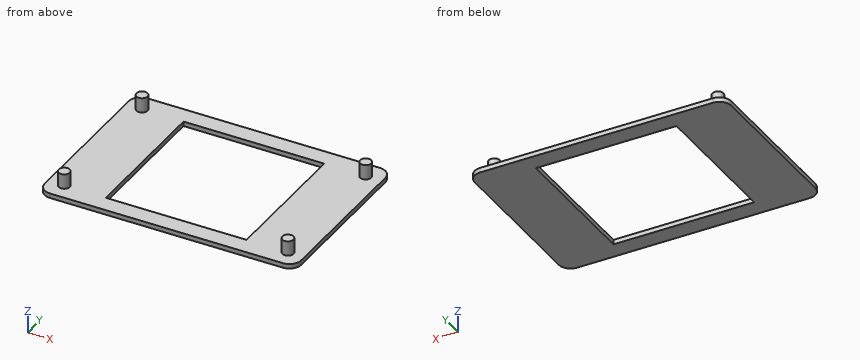
from build123d import *

# Parameters (mm, degrees)
SKETCH1_W           = 109.3978
SKETCH1_H           = 75
BOSS_EXTRUDE1_DEPTH = 2
SKETCH2_R           = 2.375
BOSS_EXTRUDE2_DEPTH = 6.35
CUT_EXTRUDE1_REACH  = 4
SKETCH3_W           = 60
SKETCH3_H           = 60
FILLET1_R           = 5


with BuildPart() as part:
    # Sketch1 → Boss-Extrude1 (new body)
    with BuildSketch(Plane.XY):
        with Locations((54.6989, 37.5)):
            Rectangle(SKETCH1_W, SKETCH1_H)
    extrude(amount=BOSS_EXTRUDE1_DEPTH)

    # Sketch2 → Boss-Extrude2 (add)
    with BuildSketch(Plane.XY.offset(2)):
        with Locations((6.9977, 67.4974)):
            Circle(SKETCH2_R)
        with Locations((102.4001, 67.4974)):
            Circle(SKETCH2_R)
        with Locations((102.4001, 7.5026)):
            Circle(SKETCH2_R)
        with Locations((6.9977, 7.5026)):
            Circle(SKETCH2_R)
    extrude(amount=BOSS_EXTRUDE2_DEPTH)

    # Sketch3 → Cut-Extrude1 (cut, up to next)
    with BuildSketch(Plane.XY.offset(2), mode=Mode.PRIVATE) as cut_extrude1_sk1:
        with Locations((54.6989, 37.5)):
            Rectangle(SKETCH3_W, SKETCH3_H)
    cut_extrude1_tool1 = extrude(cut_extrude1_sk1.sketch, amount=-CUT_EXTRUDE1_REACH, mode=Mode.PRIVATE) & part.part
    add(cut_extrude1_tool1.solids().sort_by_distance((54.6989, 37.5, 2))[0], mode=Mode.SUBTRACT)

    # Fillet1
    fillet1_edges = [part.edges().sort_by_distance(p)[0] for p in [
        (0, 75, 1),
        (109.3978, 75, 1),
        (109.3978, 0, 1),
        (0, 0, 1),
    ]]
    fillet(fillet1_edges, radius=FILLET1_R)


solid = part.part
CAD build for the part. Positions are in the model's coordinates, mm. Coordinates: 2 decimals unless noted, no trailing zeros. Write each loop counter-clockwise with the first axis right and the second up, starting at its lowest first coordinate (ties: lowest second). Pieces come first, ordered by that corner, then holes. Notation, with made-up numbers: (62.5, -0.75) - (70.5, -0.75) arc R32 ccw to (70.5, 38.25) - close; hole circle Ø5 at (14.25, 84). An arc over 180 degrees is marked (long way). Use a Markdown table: item, result. Add a question column.
Item 1: Band-saw the part on C-C, the plane x = 101.5. Give the cut face in (y, z).
Item 2: Band-saw the part on B-B, the plane x = 67. Give the cut face in (y, z), and give its area (3 significant figures).
Item 3: Flat gauge pin, fed straight in: pin 1 (5 mm diameter, centred on x = 62, z = 6, fed in from -Y). Where does the tip first touch, or does it go through?
Item 4: Band-saw the part on A-A, the plane y = 41. Give the cut face in (x, z), and give its area (3 significant figures).
Item 5: Band-saw the part on D-D, the plane z = 3.25. Give the cut face in (x, y) (3 decimals), and give its area (3 significant figures).
Item 6: Drill centre lines: L1, parallel to Y at x = 63, z = 0.5; L2, parallel to Z at x = 8, y = 46; L3, parallel to X at y = 69.5, z = 2.25. Where is each one in solid material? Low to high. Write a range as from..to.
Numbers:
| question | item | result |
|---|---|---|
| 1 | outline | (0, 0) - (75, 0) - (75, 2) - (69.7, 2) - (69.7, 8.35) - (65.3, 8.35) - (65.3, 2) - (9.7, 2) - (9.7, 8.35) - (5.3, 8.35) - (5.3, 2) - (0, 2) - close |
| 2 | outline | (0, 0) - (7.5, 0) - (7.5, 2) - (0, 2) - close; (67.5, 0) - (75, 0) - (75, 2) - (67.5, 2) - close |
| 2 | area | 30.0 mm2 |
| 3 | pin 1 | through |
| 4 | outline | (0, 0) - (24.7, 0) - (24.7, 2) - (0, 2) - close; (84.7, 0) - (109.4, 0) - (109.4, 2) - (84.7, 2) - close |
| 4 | area | 98.8 mm2 |
| 5 | outline | circle Ø4.75 at (6.998, 7.503); circle Ø4.75 at (6.998, 67.497); circle Ø4.75 at (102.4, 7.503); circle Ø4.75 at (102.4, 67.497) |
| 5 | area | 70.9 mm2 |
| 6 | L1 | 0..7.5, 67.5..75 |
| 6 | L2 | 0..2 |
| 6 | L3 | 5.72..8.27, 101.12..103.68 |
